For this review, take the finished solid that the model builds, in its own axes (mm). Give positions to 0.01 mm unless a question says otherwise; leave off trailing zeros. Loops run counter-clockwise (first coordinate to the right, second up) from the corner with the lowest first, then second, coordinate; pieces in that order, holes last. Notation, with made-up numbers: (44, 39) -> (50, 39) arc R11 ccw to (50, 59) -> close; hole circle Ø7 at (9.5, 3.5). An arc over 180 degrees is marked (long way). Answer as CSV lines item,"result". Start each with the question number.
Item 1: Add section A-A on y = 68.5. State the section outline as (x, z) points.
Item 2: Clearance check with a flat-ended pin moving along its axis: P1, Ø5, axis at x = 7.5, y = 33.5, coming from the +Z side. State where the tip first meets the part, or that it passes through.
Item 3: Add section B-B on x = -42.5. State the section outline as (y, z) points, plus the area to 3 significant figures.
Item 4: Add section C-C on z = 3.25. State how many separate pieces and enclosed holes the cut face has, plus the area to 3 significant figures.
Item 5: The part is to be moulded in two halves that separate along Y. For faces 1 (the face through (-1, -75, 5)), 2 (the face through (74, -1, 5)), 3 (the face through (39.5, -33.4, 5.1)), say which applies: +Y half, -Y half, draft (parallel to the pull), parting line (faces both ways), or undercut.
Item 6: For L1, parallel to Y at x = 12, z = 6.25; L2, parallel to Y at x = 7.5, z = 4.25; L3, parallel to X at y = -68, z = 6.75, list the stretches that pass through material, from the lowest coordinate up. Write a range as from..to.
```python
from build123d import *

# Parameters (mm, degrees)
SKETCH1_W           = 148
SKETCH1_H           = 150
BOSS_EXTRUDE1_DEPTH = 10
SKETCH2_R           = 3
SKETCH2_R_2         = 2.5
CUT_EXTRUDE1_DEPTH  = 11


with BuildPart() as part:
    # Sketch1 → Boss-Extrude1 (new body)
    with BuildSketch(Plane.XY):
        Rectangle(SKETCH1_W, SKETCH1_H)
    extrude(amount=BOSS_EXTRUDE1_DEPTH)

    # Sketch2 → Cut-Extrude1 (cut, through all)
    with BuildSketch(Plane.XY.offset(10)):
        with Locations((-42.5, 68.5)):
            Circle(SKETCH2_R)
        with Locations((-42.5, 33.5)):
            Circle(SKETCH2_R)
        with Locations((42.5, 33.5)):
            Circle(SKETCH2_R)
        with Locations((42.5, 68.5)):
            Circle(SKETCH2_R)
        with Locations((-7.5, 68.5)):
            Circle(SKETCH2_R)
        with Locations((7.5, 68.5)):
            Circle(SKETCH2_R)
        with Locations((-7.5, 33.5)):
            Circle(SKETCH2_R)
        with Locations((7.5, 33.5)):
            Circle(SKETCH2_R)
        with Locations((-12, 20)):
            Circle(SKETCH2_R_2)
        with Locations((12, 20)):
            Circle(SKETCH2_R_2)
        with Locations((12, -20)):
            Circle(SKETCH2_R_2)
        with Locations((-12, -20)):
            Circle(SKETCH2_R_2)
        with Locations((7.5, -33.5)):
            Circle(SKETCH2_R)
        with Locations((-7.5, -33.5)):
            Circle(SKETCH2_R)
        with Locations((7.5, -68.5)):
            Circle(SKETCH2_R)
        with Locations((-7.5, -68.5)):
            Circle(SKETCH2_R)
        with Locations((42.5, -68.5)):
            Circle(SKETCH2_R)
        with Locations((42.5, -33.5)):
            Circle(SKETCH2_R)
        with Locations((-42.5, -33.5)):
            Circle(SKETCH2_R)
        with Locations((-42.5, -68.5)):
            Circle(SKETCH2_R)
    extrude(amount=-CUT_EXTRUDE1_DEPTH, mode=Mode.SUBTRACT)


solid = part.part
```
Computed values:
1,outline,"(-74, 0) -> (-45.5, 0) -> (-45.5, 10) -> (-74, 10) -> close; (-39.5, 0) -> (-10.5, 0) -> (-10.5, 10) -> (-39.5, 10) -> close; (-4.5, 0) -> (4.5, 0) -> (4.5, 10) -> (-4.5, 10) -> close; (10.5, 0) -> (39.5, 0) -> (39.5, 10) -> (10.5, 10) -> close; (45.5, 0) -> (74, 0) -> (74, 10) -> (45.5, 10) -> close"
2,P1,"through"
3,outline,"(-75, 0) -> (-71.5, 0) -> (-71.5, 10) -> (-75, 10) -> close; (-65.5, 0) -> (-36.5, 0) -> (-36.5, 10) -> (-65.5, 10) -> close; (-30.5, 0) -> (30.5, 0) -> (30.5, 10) -> (-30.5, 10) -> close; (36.5, 0) -> (65.5, 0) -> (65.5, 10) -> (36.5, 10) -> close; (71.5, 0) -> (75, 0) -> (75, 10) -> (71.5, 10) -> close"
3,area,"1,260 mm²"
4,separate pieces,"1"
4,enclosed holes,"20"
4,area,"21,700 mm²"
5,face 1,"-Y half"
5,face 2,"draft"
5,face 3,"undercut"
6,L1,"-75..-22.5, -17.5..17.5, 22.5..75"
6,L2,"-75..-71.5, -65.5..-36.5, -30.5..30.5, 36.5..65.5, 71.5..75"
6,L3,"-74..-45.46, -39.54..-10.46, -4.54..4.54, 10.46..39.54, 45.46..74"
